Answer from the drawing. Dimensions are ordinates in mm from the lowest x, y and z of the part. A direction names the side the tool comes from. Coordinates: 2 decimals unless noted, no trailing zeros. Write each loop counter-clockwise with the first axis right and the second up, starting at its lowest first coordinate (ties: lowest second). Pieces come first, ordered by that corner, then holes. Notation, with made-up numbers: (82, -20) - (103, -20) arc R25 cw to (103, 16) - close; hole circle Ø9 at (55, 76). An arc over 180 degrees is marked (long way). Use a Markdown table: item, result.
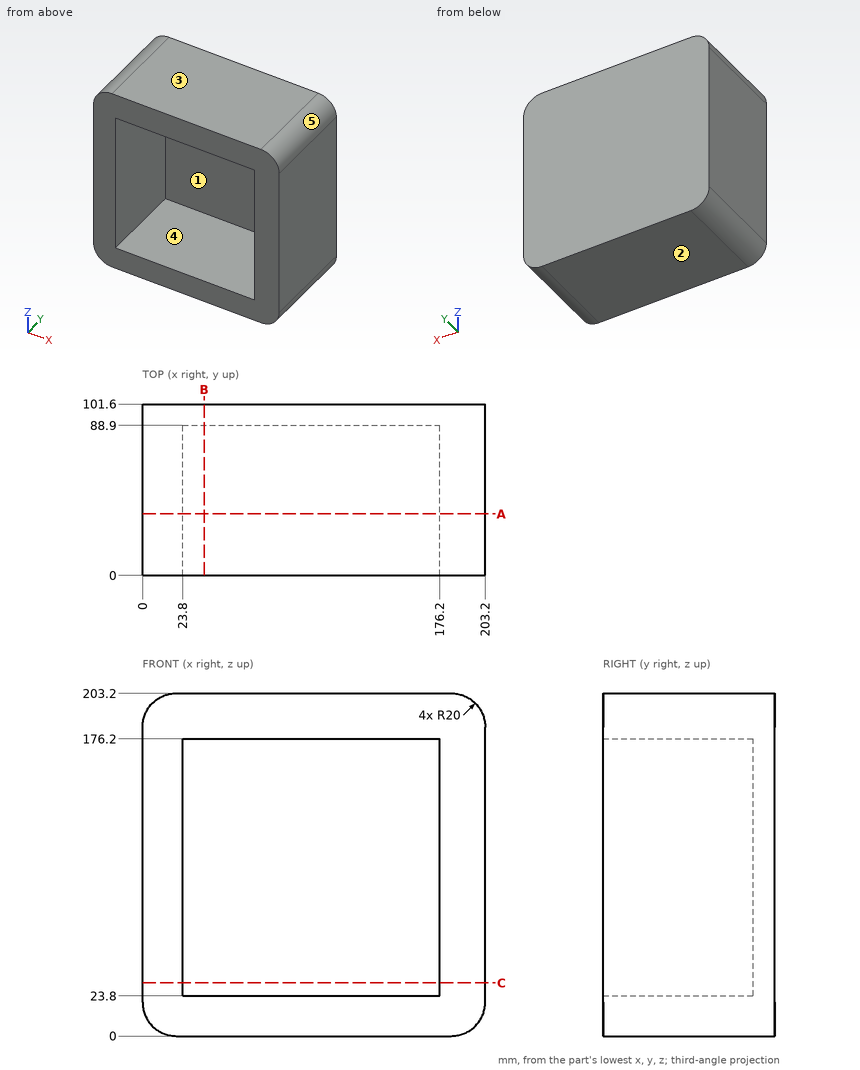
(1) The mould has two halves that part along X. Classify the marked faces 3, 4 and 5: pulls with the +X half, pulls with the -X half, needs draft (parallel to the pull), parting line crosses it, or undercut.
Report:
| item | result |
|---|---|
| face 3 | needs draft |
| face 4 | undercut |
| face 5 | pulls with the +X half |
(2) Straight lines are drawn through the part: L1, parallel to Z at x = 75, y = 18; L2, parallel to Y at x = 162, z = 66. For each, find the intervals that lie inside material, in ascending order.
Report:
| item | result |
|---|---|
| L1 | z = 0 to 23.8, 176.2 to 203.2 |
| L2 | y = 88.9 to 101.6 |
(3) Each of these flat-tipped pins is pushed along its axis until it touches: P1, Ø1, axis at y = 52.5, z = 106.5, coming from the -X side; P2, Ø1.5, axis at x = 78, z = 49, coming from the -Y side. Where does it stop, or does it pass through?
Report:
| item | result |
|---|---|
| P1 | stops at x = 0 |
| P2 | stops at y = 88.9 |
(4) A cutting plane is placed at A-A, the plane y = 36.5. Write down the section's boundary in (x, z).
Report:
| item | result |
|---|---|
| outline | (0, 20) arc R20 ccw to (20, 0) - (183.2, 0) arc R20 ccw to (203.2, 20) - (203.2, 183.2) arc R20 ccw to (183.2, 203.2) - (20, 203.2) arc R20 ccw to (0, 183.2) - close; hole (23.8, 23.8) - (176.2, 23.8) - (176.2, 176.2) - (23.8, 176.2) - close |
(5) For the marked faces 1 and 2, determine the directions among +Z, -Z, +X, -X, +Y, -Y from which every point of the face is accessible in a straight line to the end or side of a thin tool.
Report:
| item | result |
|---|---|
| face 1 | -Y |
| face 2 | -Z, +X, -X, +Y, -Y |
(6) A cutting plane is placed at B-B, the plane x = 36.5. Write down the section's boundary in (y, z), and give its area (3 significant figures).
Report:
| item | result |
|---|---|
| outline | (0, 0) - (101.6, 0) - (101.6, 203.2) - (0, 203.2) - (0, 176.2) - (88.9, 176.2) - (88.9, 23.8) - (0, 23.8) - close |
| area | 7,100 mm² |
(7) A cutting plane is placed at C-C, the plane z = 31.5. Write down the section's boundary in (x, y), and give its area (3 significant figures).
Report:
| item | result |
|---|---|
| outline | (0, 0) - (23.8, 0) - (23.8, 88.9) - (176.2, 88.9) - (176.2, 0) - (203.2, 0) - (203.2, 101.6) - (0, 101.6) - close |
| area | 7,100 mm² |
